For this review, take the finished solid that the model builds, in its own axes (mm). A direction names the side the tool comes from. Round coordinates to 2 decimals unless told otherwise and drop trailing zeros. Loops run counter-clockwise (first coordinate to the right, second up) from the corner with the lowest first, then second, coordinate; pieces in that order, holes last. Notation, with made-up numbers: M 20,-15 L 42,-15 A15 cw 42,1 Z; hole C 55.25,35 d6. An arc over 180 degrees is marked long. One line per question, with ' | ' between items. Start each with the question number.
1) Mouldability with a two-part tool opening along X and no side actions: class faces 1 (the face through (6, 10, -21)), 2 (the face through (251.15, 4.93, -151.6)), 3 (the face through (-397.117, -25.971, 236.302)) as pulls with the +X half, pulls with the -X half, needs draft (parallel to the pull), parting line crosses it, or undercut.
2) We need section C-C (y = -22). Give the boundary of the cut face in (x, z).
3) We need section A-A (x = 0). Give the boundary of the cut face in (y, z), and give its area (3 significant figures).
4) We need section B-B (z = -470). Give the boundary of the cut face in (x, y).
5) For pin 1 Ø1 at (x, z) = (153, 65.5) entering from -Y, flat-tipped, find the tip position at first contact; note if it passes through.
6) For faces 4 (the face through (-432.66, 4.93, 250.61)), 5 (the face through (3, -25.97, -479.54)), list the 3-axis set-ups (+Z, -Z, +X, -X, +Y, -Y) from which the entire face can be reached by the end or side of a thin tool; tool diameter is ignored.
7) We need section D-D (y = -80). Give the boundary of the cut face in (x, z), and give its area (3 significant figures).
8) For probe 1 along Y at (x, z) = (-149.5, -83); probe 2 along X at (y, z) = (-21, 236); probe 3 along X at (y, z) = (-68.5, 251.5), list the stretches that pass through material, from the lowest coordinate up. Write a range as from..to.
```python
from build123d import *

# Parameters (mm, degrees)
SALIENTE_EXTRUIR1_DEPTH = 10
MATRIZC1_COUNT          = 3


with BuildPart() as part:
    # Croquis1 → Saliente-Extruir1 (new body)
    with BuildSketch(Plane(origin=(0, 0, 0), x_dir=(1, 0, 0), z_dir=(0, 1, 0))):
        Polygon((-50, 500), (50, 500), (458.012701892, -206.698729811), (408.012701892, -293.301270189), (-408.012701892, -293.301270189), (-458.012701892, -206.698729811), align=None)
    extrude(amount=SALIENTE_EXTRUIR1_DEPTH)

    # Croquis2 → Revolución1 (revolve)
    with BuildSketch(Plane(origin=(0, 0, 0), x_dir=(0, 0, -1), z_dir=(1, 0, 0))):
        with BuildLine():
            Line((470, 0), (470, -70))
            Line((470, -70), (470, -90))
            ThreePointArc((470, -90), (489.318516526, -75.176380902), (480, -52.679491924))
            Line((480, -52.679491924), (480, 0))
            Line((480, 0), (470, 0))
        make_face()
    revoluci_n1 = revolve(axis=Axis((0, 0, -470), (0, -1, 0)))

    # MatrizC1: Revolución1 ×3 about axis
    matrizc1_axis = Axis((0, 0, 0), (0, 1, 0))
    for i in range(1, MATRIZC1_COUNT):
        add(revoluci_n1.rotate(matrizc1_axis, i * 360 / MATRIZC1_COUNT))


solid = part.part
```
Answers below:
1) face 1: needs draft | face 2: pulls with the +X half | face 3: undercut
2) outline: C -407.03,235 d20; C 0,-470 d20; C 407.03,235 d20
3) outline: M -52.68,-480 L 0,-480 L 0,-500 L 10,-500 L 10,293.3 L 0,293.3 L 0,-460 L -52.68,-460 A20 ccw long Z | area: 10,200 mm^2
4) outline: M -67.32,0 L -10,0 L -10,-52.68 A20 ccw long 10,-52.68 L 10,0 L 67.32,0 L 67.32,10 L -67.32,10 Z
5) pin 1: y = 0
6) face 4: +Z, -X, +Y, -Y | face 5: none
7) outline: C -407.03,235 d34.64; C 0,-470 d34.64; C 407.03,235 d34.64 | area: 2,830 mm^2
8) probe 1: 0..10 | probe 2: -416.98..-397.08, 397.08..416.98 | probe 3: -418.23..-395.83, 395.83..418.23
